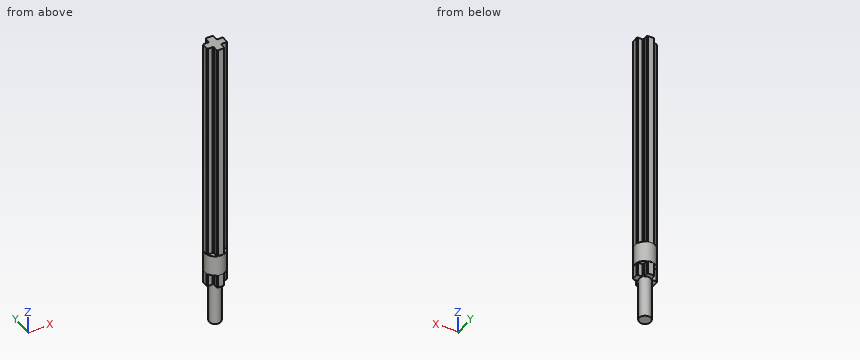
Autodesk Inventor part; units mm, degrees
ref_plane "Plano de trabajo1" through (0, 0, 0) normal (0, 0, 1) x (1, 0, 0)
ref_plane "Plano de trabajo2" through (-27.5, -25, 0) normal (0, 0, 1) x (1, 0, 0)
ref_plane "Plano de trabajo4" through (-27.5, -25, 3.2373) normal (0, 0, 1) x (1, 0, 0)
ref_plane "Plano de trabajo1" through (0, 0, 0) normal (0, 0, 1) x (1, 0, 0)
sketch "Boceto1" plane through (0, 0, 0) normal (0, 0, 1) x (1, 0, 0)
  circle A0 centre (-10, -5) radius 1.4
  point P0 (0, 0)
  dimension "d0" = 2.8
extrude "Extrusión1" add sketch "Boceto1" along normal blind 65 and the other way blind 7
sketch "Boceto3" plane through (-10, -5, 65) normal (0, 0, 1) x (1, 0, 0)
  line L0 (-2.4, 0.9) -> (2.4, 0.9)
  line L1 (2.4, 0.9) -> (2.4, -0.9)
  line L2 (2.4, -0.9) -> (-2.4, -0.9)
  line L3 (-2.4, -0.9) -> (-2.4, 0.9)
  line L4 (-2.4, 0.9) -> (2.4, -0.9) construction
  line L5 (2.4, 0.9) -> (-2.4, -0.9) construction
  circle A0 centre (0, 0) radius 1.4
  line L6 (-0.9, 2.4) -> (0.9, 2.4)
  line L7 (0.9, 2.4) -> (0.9, -2.4)
  line L8 (0.9, -2.4) -> (-0.9, -2.4)
  line L9 (-0.9, -2.4) -> (-0.9, 2.4)
  line L10 (-0.9, 2.4) -> (0.9, -2.4) construction
  line L11 (0.9, 2.4) -> (-0.9, -2.4) construction
  point P0 (10, 5)
  point P1 (0.9, 0.9)
  point P2 (-0.9, 0.9)
  point P3 (-0.9, -0.9)
  point P4 (0.9, -0.9)
  dimension "d11" = 4.8
  dimension "d12" = 1.8
ref_plane "Plano de trabajo2" through (-27.5, -25, 0) normal (0, 0, 1) x (1, 0, 0)
ref_plane "Plano de trabajo4" through (-27.5, -25, 3.2373) normal (0, 0, 1) x (1, 0, 0)
extrude "Extrusión3" add sketch "Boceto3" against normal up to surface (61.7627 mm away) contours L0 A0 L2 L3 | L0 L9 L2 A0 | L9 A0 L7 L0 | L0 L7 L2 L9 | L9 L6 L7 A0 | L0 A0 L2 L7 | L2 L7 A0 L9 | A0 L7 L8 L9 | L0 L1 L2 A0
chamfer "Chaflán1" distance 0.2 angle 45 8 edges at (-7.6, -4.1, 34.1186) (-7.6, -5.9, 34.1186) (-9.1, -7.4, 34.1186) (-10.9, -7.4, 34.1186) (-12.4, -5.9, 34.1186) (-12.4, -4.1, 34.1186) (-10.9, -2.6, 34.1186) (-9.1, -2.6, 34.1186)
ref_plane "Plano de trabajo3" through (-10, -5, 3) normal (0, 0, 1) x (0, -1, 0)
ref_plane "Plano de trabajo5" through (-22.3692, -98.1544, 6.2373) normal (0, 0, 1) x (1, 0, 0)
ref_plane "Plano de trabajo6" through (-22.3692, -98.1544, 6.2373) normal (0, 0, 1) x (1, 0, 0)
ref_plane "Plano de trabajo7" through (-10, -5, 6.4373) normal (0, 0, 1) x (0, -1, 0)
sketch "Boceto4" plane through (-10, -5, 3) normal (0, 0, 1) x (0, -1, 0)
  circle A0 centre (0, 0) radius 2.5
  point P0 (-5, 10)
  point P1 (-1.2041, 2.1909)
  dimension "d20" = 5
extrude "Extrusión4" add sketch "Boceto4" along normal blind 5 from surface at 3.4373
properties part number "EjecilindroGarraSTD"
Design review of the part built by this model. Coordinates are the model's own, in mm. Coordinates: 2 decimals unless noted, no trailing zeros. Loops run counter-clockwise (first coordinate to the right, second up) from the corner with the lowest first, then second, coordinate; pieces in that order, holes last. Notation, with made-up numbers: (60, -36.5) -> (106, -36.5) arc R6 cw to (106, -31.5) -> close; hole circle Ø11 at (25, 83). An arc over 180 degrees is marked (long way). Answer as a JSON object with one key per item and string values.
Q1. Take a section at B-B on z = 18.5. Give the boundary of the cut face in (x, y), plus the area to 3 significant figures.
Answer block:
{"outline": "(-12.4, -5.7) -> (-12.2, -5.9) -> (-11.07, -5.9) arc R1.4 ccw to (-10.9, -6.07) -> (-10.9, -7.2) -> (-10.7, -7.4) -> (-9.3, -7.4) -> (-9.1, -7.2) -> (-9.1, -6.07) arc R1.4 ccw to (-8.93, -5.9) -> (-7.8, -5.9) -> (-7.6, -5.7) -> (-7.6, -4.3) -> (-7.8, -4.1) -> (-8.93, -4.1) arc R1.4 ccw to (-9.1, -3.93) -> (-9.1, -2.8) -> (-9.3, -2.6) -> (-10.7, -2.6) -> (-10.9, -2.8) -> (-10.9, -3.93) arc R1.4 ccw to (-11.07, -4.1) -> (-12.2, -4.1) -> (-12.4, -4.3) -> close", "area": "13.9 mm^2"}
Q2. Take a section at A-A on x = -10. Give the boundary of the cut face in (y, z).
Answer block:
{"outline": "(-7.5, 6.44) -> (-7.4, 6.44) -> (-7.4, 3.24) -> (-6.4, 3.24) -> (-6.4, -7) -> (-3.6, -7) -> (-3.6, 3.24) -> (-2.6, 3.24) -> (-2.6, 6.44) -> (-2.5, 6.44) -> (-2.5, 11.44) -> (-2.6, 11.44) -> (-2.6, 65) -> (-7.4, 65) -> (-7.4, 11.44) -> (-7.5, 11.44) -> close"}
Q3. Clearance check with flat-ended pins moving along their axes: pin 1 Ø0.6 at (y, z) = (-3.5, 47) entering from +X; pin 2 Ø1.2 at (x, z) = (-12, 5.5) entering from +Y; pin 3 Ø0.6 at (y, z) = (-6.5, 30.5) entering from -X. State where each tip first meets the part, or that it passes through.
Answer block:
{"pin 1": "stops at x = -9.1", "pin 2": "stops at y = -4.1", "pin 3": "stops at x = -10.9"}
Q4. To check wall thickness, follow L1, parallel to Y at x = -11.6, z = 21; L2, parallel to X at y = -7.1, z = 47.5; L3, parallel to Y at x = -10.45, z = 52. State the ranges of each line that lie inside material, in increasing order.
Answer block:
{"L1": "y = -5.9 to -4.1", "L2": "x = -10.9 to -9.1", "L3": "y = -7.4 to -2.6"}
Q5. Take a section at C-C on y = -5. Give the boundary of the cut face in (x, z), plus the area to 3 significant figures.
Answer block:
{"outline": "(-12.5, 6.44) -> (-12.4, 6.44) -> (-12.4, 3.24) -> (-11.4, 3.24) -> (-11.4, -7) -> (-8.6, -7) -> (-8.6, 3.24) -> (-7.6, 3.24) -> (-7.6, 6.44) -> (-7.5, 6.44) -> (-7.5, 11.44) -> (-7.6, 11.44) -> (-7.6, 65) -> (-12.4, 65) -> (-12.4, 11.44) -> (-12.5, 11.44) -> close", "area": "326 mm^2"}
